```python
from build123d import *

# Parameters (mm, degrees)
F1_DEPTH = 38.1
F3_DEPTH = 25.4
F5_DEPTH = 25.4


with BuildPart() as f1:
    # F0 (on Front) → F1 (new body)
    with BuildSketch(Plane.XZ):
        Polygon((0, 12.7), (0, 0), (25.4, 0), (25.4, 31.75), (12.7, 31.75), (12.7, 12.7), align=None)
    extrude(amount=F1_DEPTH)

    # F2 (on face) → F3 (cut)
    with BuildSketch(Plane.XY.offset(12.7)):
        Polygon((0, -38.1), (12.7, -38.1), (0, -27.445292), align=None)
    extrude(amount=-F3_DEPTH, mode=Mode.SUBTRACT)

    # F4 (on face) → F5 (cut)
    with BuildSketch(Plane(origin=(12.7, 0, 0), x_dir=(0, -1, 0), z_dir=(-1, 0, 0))):
        Polygon((27.73655, 31.75), (38.1, 18.929737), (38.1, 31.75), align=None)
    extrude(amount=-F5_DEPTH, mode=Mode.SUBTRACT)


solid = f1.part
```
Could you check a few things on this model? Use its own coordinates, in mm. A direction names the side the tool comes from. Round coordinates to 2 decimals unless told otherwise and drop trailing zeros. Order: outer loops, then holes, each group sorted by start corner. A loop starts at its lowest first (then second) coordinate and runs counter-clockwise, first axis right, second up. Notation, with made-up numbers: (32, 57.5) -> (57, 57.5) arc R29 ccw to (57, 86.5) -> close; hole circle Ø6 at (18, -6.5). An arc over 180 degrees is marked (long way). One line per question, with ' | ' between items.
Q1. If we section it at A-A on x = 14.5: Write out the boundary of the cut face in (y, z).
Computed values:
outline: (-38.1, 0) -> (0, 0) -> (0, 31.75) -> (-27.74, 31.75) -> (-38.1, 18.93) -> close
Q2. I'm going to push flat-ended pins straight in: pin 1 (1 mm diameter, centred on x = 17, y = -32.5, fed in from +Z); pin 2 (1 mm diameter, centred on x = 4, y = -20, fed in from +Z); pin 3 (1.5 mm diameter, centred on x = 16, z = 25, fed in from -Y). Where does each tip first touch, or does it pass through?
Computed values:
pin 1: z = 26.48 | pin 2: z = 12.7 | pin 3: y = -33.8
Q3. If we section it at B-B on z = 3: Write out the boundary of the cut face in (x, y), plus the area to 3 significant figures.
Computed values:
outline: (0, -27.45) -> (12.7, -38.1) -> (25.4, -38.1) -> (25.4, 0) -> (0, 0) -> close | area: 900 mm²
Q4. If I drill on line 1 (X direction, y = -25.5, z = 22.5); line 2 (Z direction, x = 9.5, y = -29); line 3 (Y direction, x = 5.25, z = 3), over which ranges is the centre line in solid material (lowest first)? Write a range as from..to.
Computed values:
line 1: 12.7..25.4 | line 2: 0..12.7 | line 3: -31.85..0
Q5. If we section it at D-D on y = -33.5: Write out the boundary of the cut face in (x, z).
Computed values:
outline: (7.22, 0) -> (25.4, 0) -> (25.4, 24.62) -> (12.7, 24.62) -> (12.7, 12.7) -> (7.22, 12.7) -> close
Q6. Which directions (+Z, -Z, +X, -X, +Y, -Y) give clear straight access to the entire face, cutting with the end or side of a thin tool? Please do faces 1 (the face through (12.7, -19, 22)), 2 (the face through (19, -14, 31.75)).
Computed values:
face 1: +Z, -X, +Y, -Y | face 2: +Z, +X, -X, +Y, -Y
Q7. If we section it at C-C on y = -24: Write out the boundary of the cut face in (x, z), plus the area to 3 significant figures.
Computed values:
outline: (0, 0) -> (25.4, 0) -> (25.4, 31.75) -> (12.7, 31.75) -> (12.7, 12.7) -> (0, 12.7) -> close | area: 565 mm²
